from build123d import *

# Parameters (mm, degrees)
BOSS_EXTRUDE1_DEPTH = 8
SKETCH2_R           = 6
SKETCH2_R_2         = 3
SKETCH2_R_3         = 3.15
CUT_EXTRUDE1_DEPTH  = 4
SKETCH3_R           = 5
CUT_EXTRUDE2_DEPTH  = 10
SKETCH4_R           = 3.15
CUT_EXTRUDE4_DEPTH  = 11


with BuildPart() as part:
    # Sketch1 → Boss-Extrude1 (new body)
    with BuildSketch(Plane(origin=(0, 0, 0), x_dir=(1, 0, 0), z_dir=(0, 1, 0))):
        with BuildLine():
            Line((12.990381057, 22.5), (34.607695155, 59.942286341))
            ThreePointArc((34.607695155, 59.942286341), (45, 65.942286341), (55.392304845, 59.942286341))
            Line((55.392304845, 59.942286341), (77.009618943, 22.5))
            ThreePointArc((77.009618943, 22.5), (77.009618943, 7.5), (64.019237886, 0))
            Line((64.019237886, 0), (25.980762114, 0))
            ThreePointArc((25.980762114, 0), (12.990381057, 7.5), (12.990381057, 22.5))
        make_face()
    extrude(amount=BOSS_EXTRUDE1_DEPTH)

    # Sketch2 → Cut-Extrude1 (cut)
    with BuildSketch(Plane(origin=(0, 8, 0), x_dir=(1, 0, 0), z_dir=(0, 1, 0))):
        with Locations((45, 54.358166274)):
            Circle(SKETCH2_R)
        with Locations((30, 10)):
            Circle(SKETCH2_R_2)
        with Locations((60, 10)):
            Circle(SKETCH2_R_3)
    extrude(amount=-CUT_EXTRUDE1_DEPTH, mode=Mode.SUBTRACT)

    # Sketch3 → Cut-Extrude2 (cut)
    with BuildSketch(Plane(origin=(0, 4, 0), x_dir=(1, 0, 0), z_dir=(0, 1, 0))):
        with Locations((45, 54.358166274)):
            Circle(SKETCH3_R)
    extrude(amount=-CUT_EXTRUDE2_DEPTH, mode=Mode.SUBTRACT)

    # Sketch4 → Cut-Extrude4 (cut)
    with BuildSketch(Plane(origin=(0, 0, 0), x_dir=(1, 0, 0), z_dir=(0, 1, 0))):
        with Locations((30, 10)):
            Circle(SKETCH4_R)
        with Locations((60, 10)):
            Circle(SKETCH4_R)
    extrude(amount=CUT_EXTRUDE4_DEPTH, mode=Mode.SUBTRACT)


solid = part.part
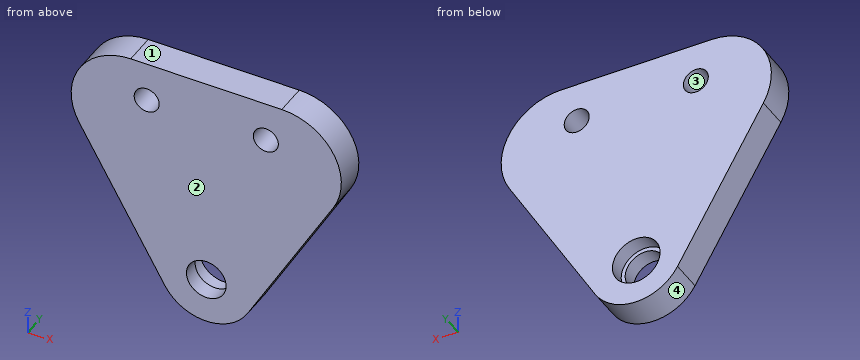
Source: CAD feature listing. Evaluate the final solid. Frame: model axes, mm. Face numbers are marked on the shaded views. Round coordinates to 2 decimals unless told otherwise and drop trailing zeros. Loops run counter-clockwise (first coordinate to the right, second up) from the corner with the lowest first, then second, coordinate; pieces in that order, holes last. Notation, with made-up numbers: (77, 69) -> (124, 69) arc R18 cw to (124, 82) -> close; hole circle Ø4 at (67.5, -13.5). An arc over 180 degrees is marked (long way). Answer as a JSON object with one key per item and string values. Group by question number.
Q1. Section query A-A (x = 45). Output: boundary loops of the cut face in (y, z), plus the area to 3 significant figures.
Q2. Ray query, line 1 (X direction, y = 2, z = -10); line 2 (Z direction, x = 45, y = 3.2); line 3 (Z direction, x = 60, y = 1.75). Return the intervals inside material, ascending. Write a range as from..to.
Q3. Section query C-C (z = -10). Output: boundary loops of the cut face in (x, y).
Q4. Mould query, pull axis Z, two halves, no side actions, for the marked faces 1, 2, 3 and 4. Classes: pulls with the +Z half, pulls with the -Z half, needs draft (parallel to the pull), parting line crosses it, or undercut.
Q5. Contact query for flat-ended pins moving along their axis: P1, Ø13, axis at x = 44.5, z = -55.5, coming from the +Y side; P2, Ø2, axis at y = 2, z = -54.5, coming from the +X side; P3, Ø1, axis at x = 69, y = 4, coming from the -Z side. Output: stop coordinate, or through.
Q6. Section query D-D (z = -57.5). Output: boundary loops of the cut face in (x, y), plus the area to 3 significant figures.
Q7. Section query B-B (y = 6.5). Output: boundary loops of the cut face in (x, z).
Completed:
{
 "1": {"outline": "(0, -65.94) -> (8, -65.94) -> (8, -60.36) -> (4, -60.36) -> (4, -59.36) -> (0, -59.36) -> close; (0, -49.36) -> (4, -49.36) -> (4, -48.36) -> (8, -48.36) -> (8, 0) -> (0, 0) -> close", "area": "440 mm²"},
 "2": {"line 1": "11.84..26.85, 33.15..56.85, 63.15..78.16", "line 2": "-65.94..-59.36, -49.36..0", "line 3": "-51.96..-13.15, -6.85..0"},
 "3": {"outline": "(11.84, 0) -> (26.85, 0) -> (26.85, 8) -> (11.84, 8) -> close; (33.15, 0) -> (56.85, 0) -> (56.85, 8) -> (33.15, 8) -> close; (63.15, 0) -> (78.16, 0) -> (78.16, 8) -> (63.15, 8) -> close"},
 "4": {"face 1": "pulls with the +Z half", "face 2": "needs draft", "face 3": "undercut", "face 4": "pulls with the -Z half"},
 "5": {"P1": "y = 8", "P2": "x = 59.11", "P3": "z = -37.24"},
 "6": {"outline": "(33.2, 0) -> (41.11, 0) -> (41.11, 4) -> (39.89, 4) -> (39.89, 8) -> (33.2, 8) -> close; (48.89, 0) -> (56.8, 0) -> (56.8, 8) -> (50.11, 8) -> (50.11, 4) -> (48.89, 4) -> close", "area": "117 mm²"},
 "7": {"outline": "(12.99, -22.5) -> (34.61, -59.94) arc R12 ccw to (55.39, -59.94) -> (77.01, -22.5) arc R15 ccw to (64.02, 0) -> (25.98, 0) arc R15 ccw to start; hole circle Ø6.3 at (30, -10); hole circle Ø12 at (45, -54.36); hole circle Ø6.3 at (60, -10)"}
}
